Can you work these out from the drawing? Everything is in mm from the part's minimum corner. A direction names the side the tool comes from. Round coordinates to 2 decimals unless told otherwise and drop trailing zeros. Loops run counter-clockwise (first coordinate to the right, second up) from the corner with the lowest first, then second, coordinate; pieces in that order, holes last. Notation, with made-up numbers: (-6, -2) -> (26, -2) arc R34 ccw to (26, 32) -> close; hole circle Ø7 at (80, -26). An arc over 180 degrees is marked (long way). Answer as a JSON object with one key per item and string values.
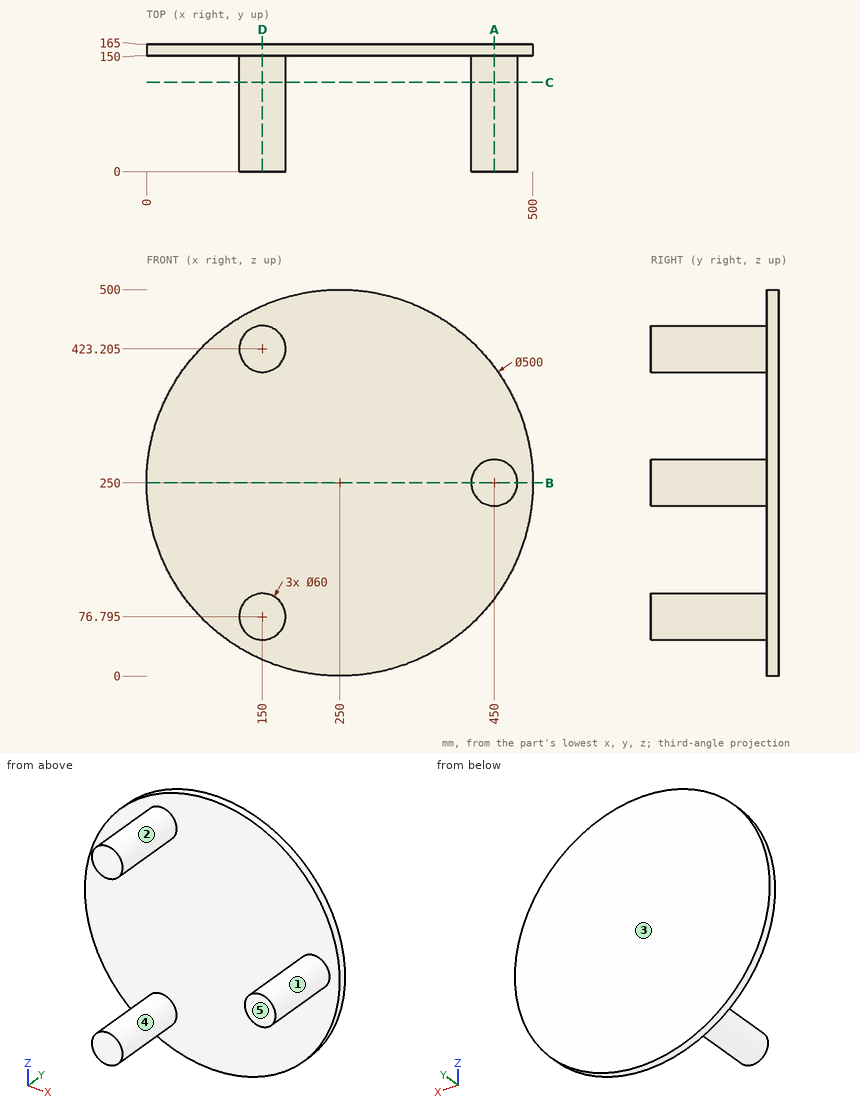
Q1. I'm going to push flat-ended pins straight in: pin 1 (12 mm diameter, centred on y = 102.5, z = 426, fed in from -X); pin 2 (5 mm diameter, centred on x = 254, z = 266, fed in from -Y); pin 3 (8 mm diameter, centred on x = 147, y = 104, fed in from +Z) (3 decimals). Where does each tip first touch, or does it pass through?
Determined:
{"pin 1": "x = 120", "pin 2": "y = 150", "pin 3": "z = 453.205"}
Q2. I want a section at C-C, the plane y = 115.5. Write out the boundary of the cut face in (x, z) (3 decimals), then the cut area to 3 significant figures.
Determined:
{"outline": "circle Ø60 at (150, 76.795); circle Ø60 at (150, 423.205); circle Ø60 at (450, 250)", "area": "8,480 mm²"}
Q3. On a 3-axis mill with a long thin cutter (end or side, diameter ignored), from which of +Z, -Z, +X, -X, +Y, -Y can I reach the whole of each face in a straight line? I mean the marked faces 4 and 5. Say none if no direction works.
Determined:
{"face 4": "-Y", "face 5": "+Z, -Z, +X, -X, -Y"}
Q4. I want a section at D-D, the plane x = 150. Write out the boundary of the cut face in (y, z) (3 decimals).
Determined:
{"outline": "(0, 46.795) -> (150, 46.795) -> (150, 20.871) -> (165, 20.871) -> (165, 479.129) -> (150, 479.129) -> (150, 453.205) -> (0, 453.205) -> (0, 393.205) -> (150, 393.205) -> (150, 106.795) -> (0, 106.795) -> close"}
Q5. I want a section at B-B, the plane z = 250. Write out the boundary of the cut face in (x, y).
Determined:
{"outline": "(0, 150) -> (420, 150) -> (420, 0) -> (480, 0) -> (480, 150) -> (500, 150) -> (500, 165) -> (0, 165) -> close"}
Q6. I want a section at A-A, the plane x = 450. Write out the boundary of the cut face in (y, z), then the cut area to 3 significant figures.
Determined:
{"outline": "(0, 220) -> (150, 220) -> (150, 100) -> (165, 100) -> (165, 400) -> (150, 400) -> (150, 280) -> (0, 280) -> close", "area": "13,500 mm²"}
Q7. If I drill on L1, parallel to Y at x = 302.5, z = 409.5; L2, parallel to X at y = 27, z = 412; L3, parallel to X at y = 97, z = 264.5, over which ranges is the centre line in solid material (lowest first)? Write a range as [from, to].
Determined:
{"L1": "[150, 165]", "L2": "[122.17, 177.83]", "L3": "[423.74, 476.26]"}
Q8. We'd pull the mould along Z, two halves only. Please class the marked faces 1, 2 and 3: pulls with the +Z half, pulls with the -Z half, needs draft (parallel to the pull), parting line crosses it, or undercut.
Determined:
{"face 1": "parting line crosses it", "face 2": "undercut", "face 3": "needs draft"}
